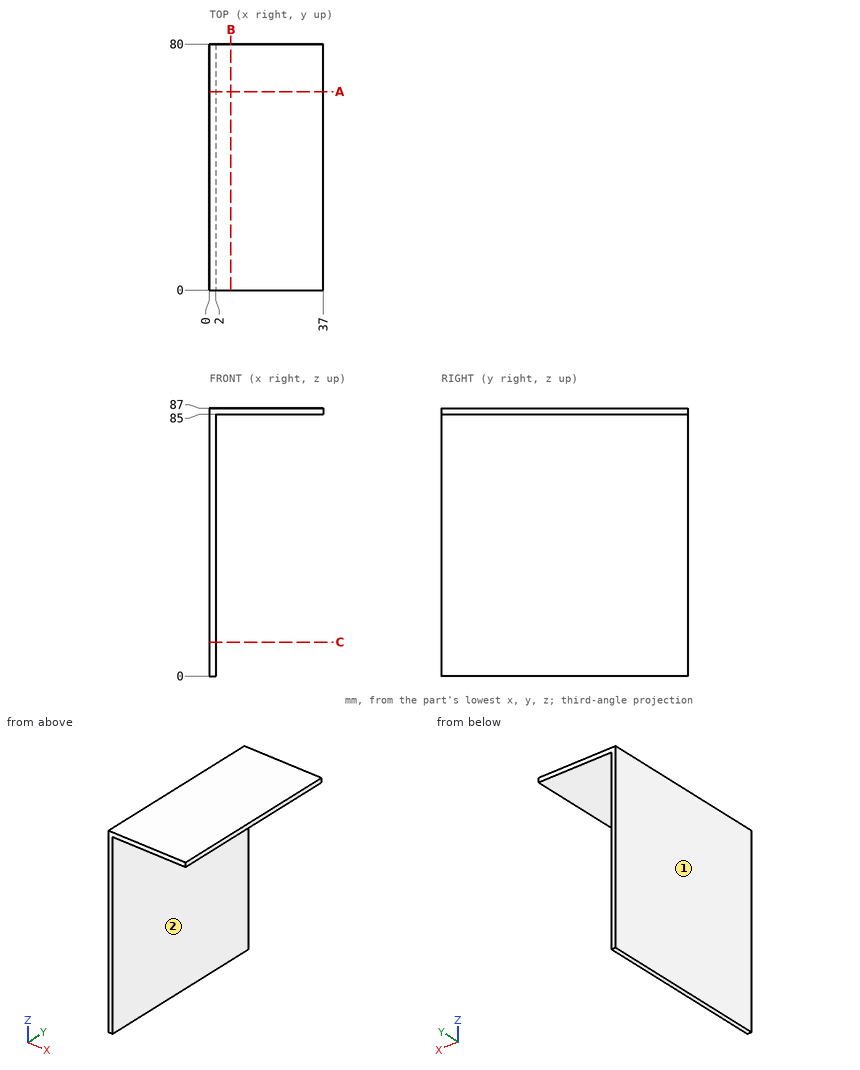
Study the drawing (mm; zero at the part's minimum x, y, z) and answer. A direction names the side the tool comes from. Coordinates: 2 decimals unless noted, no trailing zeros. Loops run counter-clockwise (first coordinate to the right, second up) from the corner with the lowest first, then second, coordinate; pieces in that order, holes last. Notation, with made-up numbers: (59.5, 71.5) -> (114.5, 71.5) arc R21 ccw to (114.5, 75.5) -> close; hole circle Ø6 at (84, 10.25). An arc over 180 degrees is marked (long way). Write item = value, one per line. Start each with the question number.
1) The part is cut by section A-A, the plane y = 64.5. Determine the outline of the cut face in (x, z).
2) The part is cut by section B-B, the plane x = 7. Determine the outline of the cut face in (y, z), plus the area to 3 significant figures.
3) Find the intervals of material crossed by L1, parallel to Z at x = 18.5, y = 12; L2, parallel to X at y = 70, z = 72.5, in increasing order. Write a range as from..to.
4) Given P1, Ø4, axis at y = 37.5, z = 35.5, coming from the -X side; P2, Ø3, axis at x = 13, y = 44.5, coming from the -Z side; P3, Ø6, axis at y = 53.5, z = 20.5, coming from the +X side, each flat-ended and moving along its own axis, determine where each tip first touches the part or whether it passes through.
5) The part is cut by section C-C, the plane z = 11. Determine the outline of the cut face in (x, y), plus the area to 3 significant figures.
6) For the marked faces 1 and 2, determine the directions among +Z, -Z, +X, -X, +Y, -Y from which every point of the face is accessible in a straight line to the end or side of a thin tool.
Result:
q1.outline = (0, 0) -> (2, 0) -> (2, 85) -> (37, 85) -> (37, 87) -> (0, 87) -> close
q2.outline = (0, 85) -> (80, 85) -> (80, 87) -> (0, 87) -> close
q2.area = 160 mm²
q3.L1 = 85..87
q3.L2 = 0..2
q4.P1 = 0
q4.P2 = 85
q4.P3 = 2
q5.outline = (0, 0) -> (2, 0) -> (2, 80) -> (0, 80) -> close
q5.area = 160 mm²
q6.face_1 = +Z, -Z, -X, +Y, -Y
q6.face_2 = -Z, +X, +Y, -Y
